Autodesk Inventor part; units mm, degrees
ref_plane "YZ Plane" through (0, 0, 0) normal (1, 0, 0) x (0, 1, 0)
ref_plane "XZ Plane" through (0, 0, 0) normal (0, 1, 0) x (-1, 0, 0)
ref_plane "XY Plane" through (0, 0, 0) normal (0, 0, 1) x (1, 0, 0)
sketch "Sketch1" plane through (0, 0, 0) normal (0, 0, 1) x (1, 0, 0)
  line L0 (0, 0) -> (50.8, 0)
  line L1 (50.8, 0) -> (50.8, 50.8)
  line L2 (50.8, 50.8) -> (0, 50.8)
  line L3 (0, 50.8) -> (0, 0)
  line L4 (0, 0) -> (4.7625, 0) construction
  line L5 (4.7625, 0) -> (4.7625, 4.7625) construction
  line L6 (4.7625, 4.7625) -> (0, 4.7625) construction
  line L7 (0, 4.7625) -> (0, 0) construction
  line L8 (50.8, 50.8) -> (46.0375, 50.8) construction
  line L9 (46.0375, 50.8) -> (46.0375, 46.0375) construction
  line L10 (46.0375, 46.0375) -> (50.8, 46.0375) construction
  line L11 (50.8, 46.0375) -> (50.8, 50.8) construction
  line L12 (46.0375, 46.0375) -> (4.7625, 46.0375)
  line L13 (4.7625, 46.0375) -> (4.7625, 4.7625)
  line L14 (4.7625, 4.7625) -> (46.0375, 4.7625)
  line L15 (46.0375, 4.7625) -> (46.0375, 46.0375)
  dimension "d0" = 50.8
  dimension "d1" = 50.8
  dimension "d2" = 4.7625
  dimension "d3" = 4.7625
  dimension "d4" = 4.7625
  dimension "d5" = 4.7625
extrude "Extrusion1" add sketch "Sketch1" along normal blind 1016
equation "\"d0\" = d1"
equation "\"d2\" = d3"
equation "\"d4\" = d3"
equation "\"d5\" = d3"
properties part number "40in2.0Sq" material "Steel, Mild"
Can you work these out from the model? Positions are in its coordinate system, mm. A direction names the side the tool comes from. Round coordinates to 2 decimals unless told otherwise and drop trailing zeros. Loops run counter-clockwise (first coordinate to the right, second up) from the corner with the lowest first, then second, coordinate; pieces in that order, holes last. Notation, with made-up numbers: (69, -20.75) -> (82, -20.75) arc R34 cw to (82, 9.25) -> close; hole circle Ø1 at (31, -9.75). An arc over 180 degrees is marked (long way). One line per item, written item: value. Start each with the question number.
1. If we section it at A-A, the plane y = 17: Write out the boundary of the cut face in (x, z), then the cut area to 3 significant figures.
2. For faces 5 (the flat face through (0, 26, 501)), 6 (the flat face through (26, 46.038, 501)), which set-ups out of +Z, -Z, +X, -X, +Y, -Y let a thin tool reach every point of the face, with its end or its side?
3. For pin 1 (12.5 mm diameter, centred on x = 28.5, z = 548, fed in from -Y), with a flat end and sliding along its axis, tell me the tip position at first contact or that it passes through.
4. If I drill on probe 1 along X at (y, z) = (45.5, 876), over which ranges is the centre line in solid material (lowest first)?
5. If we mould it in two halves opening along Y, with no side actions, what happens to faces 1 (the flat face through (26, 50.8, 501)), 2 (the flat face through (25, 0, 501)), 3 (the flat face through (46.038, 25, 501)), 4 (the flat face through (25, 4.762, 501))? For each: pulls with the +Y half, pulls with the -Y half, needs draft (parallel to the pull), parting line crosses it, or undercut.
6. If we section it at C-C, the plane z = 546.5: Write out the boundary of the cut face in (x, y), then the cut area to 3 significant figures.
Calculated:
1. outline: (0, 0) -> (4.76, 0) -> (4.76, 1016) -> (0, 1016) -> close; (46.04, 0) -> (50.8, 0) -> (50.8, 1016) -> (46.04, 1016) -> close
1. area: 9,680 mm²
2. face 5: +Z, -Z, -X, +Y, -Y
2. face 6: +Z, -Z
3. pin 1: stops at y = 0
4. probe 1: x = 0 to 4.76, 46.04 to 50.8
5. face 1: pulls with the +Y half
5. face 2: pulls with the -Y half
5. face 3: undercut
5. face 4: undercut
6. outline: (0, 0) -> (50.8, 0) -> (50.8, 50.8) -> (0, 50.8) -> close; hole (4.76, 4.76) -> (46.04, 4.76) -> (46.04, 46.04) -> (4.76, 46.04) -> close
6. area: 877 mm²
